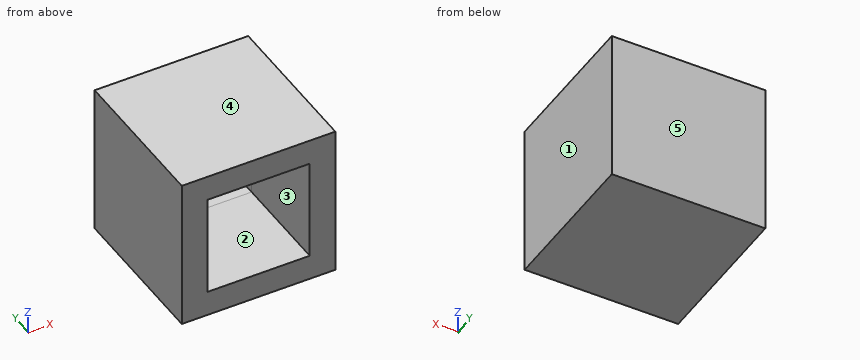
```python
from build123d import *

# Parameters (mm, degrees)
F0_W     = 30
F0_H     = 30
F1_DEPTH = 30
F2_T     = -5
F3_R     = 5


with BuildPart() as f1:
    # F0 (on Front) → F1 (new body)
    with BuildSketch(Plane.XZ):
        with Locations((15, 15)):
            Rectangle(F0_W, F0_H)
    extrude(amount=F1_DEPTH)

    # F2
    f2_openings = [f1.faces().sort_by_distance(p)[0] for p in [
        (15, -30, 15),
    ]]
    offset(amount=F2_T, openings=f2_openings)

    # F3
    f3_edges = [f1.edges().sort_by_distance(p)[0] for p in [
        (5, -5, 15),
        (15, -5, 5),
        (25, -5, 15),
        (15, -5, 25),
    ]]
    fillet(f3_edges, radius=F3_R)


solid = f1.part
```
Design review of the part built by this model. Coordinates are the model's own, in mm. Face numbers are marked on the shaded views. A direction names the side the tool comes from. Coordinates: 2 decimals unless noted, no trailing zeros. Order: outer loops, then holes, each group sorted by start corner. A loop starts at its lowest first (then second) coordinate and runs counter-clockwise, first axis right, second up. Notation, with made-up numbers: (6.5, 62) - (58.5, 62) arc R20 ccw to (58.5, 97) - close; hole circle Ø4 at (20.5, -25.5). An arc over 180 degrees is marked (long way). Answer in a Markdown table with one row per item.
(1) Consider section D-D on y = -6.5. State the section outline as (x, z) points, plus the area to 3 significant figures.
Checked values:
| item | result |
|---|---|
| outline | (0, 0) - (30, 0) - (30, 30) - (0, 30) - close; hole (6.43, 6.43) - (23.57, 6.43) - (23.57, 23.57) - (6.43, 23.57) - close |
| area | 606 mm^2 |
(2) Consider section A-A on y = -20.75. State the section outline as (x, z) points, plus the area to 3 significant figures.
Checked values:
| item | result |
|---|---|
| outline | (0, 0) - (30, 0) - (30, 30) - (0, 30) - close; hole (5, 5) - (25, 5) - (25, 25) - (5, 25) - close |
| area | 500 mm^2 |
(3) For the marked faces 1 and 2, list the 3-axis set-ups (+Z, -Z, +X, -X, +Y, -Y) from which the entire face can be reached by the end or side of a thin tool; tool diameter is ignored.
Checked values:
| item | result |
|---|---|
| face 1 | +Z, -Z, +X, +Y, -Y |
| face 2 | -Y |
(4) Wall thickness on line 1 along X through (y, z) = (-18, 5.25); line 2 along Z through (x, y) = (13, -6.5): over which ranges is each line inside the solid? List them lowest first. Write a range as from..to.
Checked values:
| item | result |
|---|---|
| line 1 | 0..5, 25..30 |
| line 2 | 0..6.43, 23.57..30 |
(5) Consider section C-C on x = 14. State the section outline as (y, z) points, plus the area to 3 significant figures.
Checked values:
| item | result |
|---|---|
| outline | (-30, 0) - (0, 0) - (0, 30) - (-30, 30) - (-30, 25) - (-10, 25) arc R5 cw to (-5, 20) - (-5, 10) arc R5 cw to (-10, 5) - (-30, 5) - close |
| area | 411 mm^2 |
(6) The part is to be moulded in two halves that separate along Z. For the marked faces 3, 4 and 5, say which applies: released by +Z, released by -Z, zero draft, split by the parting line, or undercut.
Checked values:
| item | result |
|---|---|
| face 3 | undercut |
| face 4 | released by +Z |
| face 5 | zero draft |
(7) Consider section B-B on z = 17.5. State the section outline as (x, y) points, plus the area to 3 significant figures.
Checked values:
| item | result |
|---|---|
| outline | (0, -30) - (5, -30) - (5, -10) arc R5 cw to (10, -5) - (20, -5) arc R5 cw to (25, -10) - (25, -30) - (30, -30) - (30, 0) - (0, 0) - close |
| area | 411 mm^2 |
(8) Clearance check with a flat-ended pin moving along its axis: pin 1 (5 mm diameter, centred on x = 14, z = 17.5, fed in from -Y). State where the tip first meets the part, or that it passes through.
Checked values:
| item | result |
|---|---|
| pin 1 | y = -5 |
